Can you work these out from the model? Positions are in its coordinate system, mm. A direction names the side the tool comes from. Round coordinates to 2 decimals unless told otherwise and drop trailing zeros. Loops run counter-clockwise (first coordinate to the right, second up) from the corner with the lowest first, then second, coordinate; pieces in that order, holes last. Notation, with made-up numbers: (1, -18.5) -> (17, -18.5) arc R25 cw to (17, 15.5) -> close; hole circle Ø3 at (30, 18). An arc over 180 degrees is marked (long way). Answer as a JSON object with one key per item and string values.
```python
from build123d import *

# Parameters (mm, degrees)
F0_R      = 36.25
F1_DEPTH  = 17
F2_R      = 32.25
F3_DEPTH  = 4
F4_R      = 1.5
F5_DEPTH  = 15
F7_R      = 2
F8_DEPTH  = 25
F10_R     = 2
F11_DEPTH = 25
F13_DEPTH = 12


with BuildPart() as f1:
    # F0 (on Front) → F1 (new body)
    with BuildSketch(Plane.XZ):
        Circle(F0_R)
        with BuildLine():
            Line((-33, -99), (-18.995849, -99))
            Line((-18.995849, -99), (0, -99))
            Line((0, -99), (18.995849, -99))
            Line((18.995849, -99), (33, -79))
            Line((33, -79), (33, -37.56328))
            ThreePointArc((33, -37.56328), (45.552168, -20.615528), (50, 0))
            ThreePointArc((50, 0), (45.552168, 20.615528), (33, 37.56328))
            Line((33, 37.56328), (33, 79))
            Line((33, 79), (18.995849, 99))
            Line((18.995849, 99), (-18.995849, 99))
            Line((-18.995849, 99), (-33, 99))
            Line((-33, 99), (-33, 79))
            Line((-33, 79), (-33, 37.56328))
            ThreePointArc((-33, 37.56328), (-45.552168, 20.615528), (-50, 0))
            ThreePointArc((-50, 0), (-45.552168, -20.615528), (-33, -37.56328))
            Line((-33, -37.56328), (-33, -79))
            Line((-33, -79), (-33, -99))
        make_face()
        Circle(F0_R, mode=Mode.SUBTRACT)
    extrude(amount=F1_DEPTH)

    # F2 (on face) → F3 (join)
    with BuildSketch(Plane.XZ.offset(17)):
        with BuildLine():
            Line((33, -79), (33, -37.56328))
            ThreePointArc((33, -37.56328), (50, 0), (33, 37.56328))
            Line((33, 37.56328), (33, 79))
            Line((33, 79), (18.995849, 99))
            Line((18.995849, 99), (-33, 99))
            Line((-33, 99), (-33, 37.56328))
            ThreePointArc((-33, 37.56328), (-50, 0), (-33, -37.56328))
            Line((-33, -37.56328), (-33, -99))
            Line((-33, -99), (18.995849, -99))
            Line((18.995849, -99), (33, -79))
        make_face()
        Circle(F2_R, mode=Mode.SUBTRACT)
    extrude(amount=F3_DEPTH)

    # F4 (on face) → F5 (cut)
    with BuildSketch(Plane(origin=(0, 0, 0), x_dir=(-1, 0, 0), z_dir=(0, 1, 0))):
        with Locations((-18, -42.60355)):
            Circle(F4_R)
        with Locations((18, -42.60355)):
            Circle(F4_R)
        with Locations((18, -67.60355)):
            Circle(F4_R)
        with Locations((-18, -67.60355)):
            Circle(F4_R)
    extrude(amount=-F5_DEPTH, mode=Mode.SUBTRACT)

    # F7 (on offset) → F8 (cut)
    with BuildSketch(Plane.YZ.offset(21)):
        with BuildLine():
            ThreePointArc((-12.5, -85.60355), (-10.5, -87.60355), (-8.5, -85.60355))
            Line((-8.5, -85.60355), (-12.5, -85.60355))
        make_face()
        with BuildLine():
            Line((-12.5, -85.60355), (-8.5, -85.60355))
            ThreePointArc((-8.5, -85.60355), (-10.5, -83.60355), (-12.5, -85.60355))
        make_face()
        with BuildLine():
            ThreePointArc((-12.5, -55.10355), (-10.5, -57.10355), (-8.5, -55.10355))
            Line((-8.5, -55.10355), (-12.5, -55.10355))
        make_face()
        with BuildLine():
            Line((-12.5, -55.10355), (-8.5, -55.10355))
            ThreePointArc((-8.5, -55.10355), (-10.5, -53.10355), (-12.5, -55.10355))
        make_face()
        with Locations((-10.5, 55.10355)):
            Circle(F7_R)
        with Locations((-10.5, 85.60355)):
            Circle(F7_R)
    extrude(amount=F8_DEPTH, mode=Mode.SUBTRACT)

    # F10 (on offset) → F11 (cut)
    with BuildSketch(Plane.YZ.offset(-21)):
        with BuildLine():
            ThreePointArc((-12.5, -85.60355), (-10.5, -87.60355), (-8.5, -85.60355))
            Line((-8.5, -85.60355), (-12.5, -85.60355))
        make_face()
        with BuildLine():
            Line((-12.5, -85.60355), (-8.5, -85.60355))
            ThreePointArc((-8.5, -85.60355), (-10.5, -83.60355), (-12.5, -85.60355))
        make_face()
        with BuildLine():
            ThreePointArc((-12.5, -55.10355), (-10.5, -57.10355), (-8.5, -55.10355))
            Line((-8.5, -55.10355), (-12.5, -55.10355))
        make_face()
        with BuildLine():
            Line((-12.5, -55.10355), (-8.5, -55.10355))
            ThreePointArc((-8.5, -55.10355), (-10.5, -53.10355), (-12.5, -55.10355))
        make_face()
        with Locations((-10.5, 55.10355)):
            Circle(F10_R)
        with Locations((-10.5, 85.60355)):
            Circle(F10_R)
    extrude(amount=-F11_DEPTH, mode=Mode.SUBTRACT)

    # F12 (on face) → F13 (cut)
    with BuildSketch(Plane(origin=(0, 0, 0), x_dir=(-1, 0, 0), z_dir=(0, 1, 0))):
        with BuildLine():
            ThreePointArc((0, -87.25), (-2, -89.25), (0, -91.25))
            Line((0, -91.25), (0, -87.25))
        make_face()
        with BuildLine():
            Line((0, -87.25), (0, -91.25))
            ThreePointArc((0, -91.25), (1.414214, -90.664214), (2, -89.25))
            ThreePointArc((2, -89.25), (1.414214, -87.835786), (0, -87.25))
        make_face()
    extrude(amount=-F13_DEPTH, mode=Mode.SUBTRACT)


solid = f1.part
```
Q1. I want a section at D-D, the plane x = 40. Write out the boundary of the cut face in (y, z).
Determined:
{"outline": "(-21, -30) -> (0, -30) -> (0, 30) -> (-21, 30) -> close"}
Q2. I want a section at B-B, the plane z = -20. Write out the boundary of the cut face in (x, y), then the cut area to 3 significant figures.
Determined:
{"outline": "(-45.83, -21) -> (-25.3, -21) -> (-25.3, -17) -> (-30.23, -17) -> (-30.23, 0) -> (-45.83, 0) -> close; (25.3, -21) -> (45.83, -21) -> (45.83, 0) -> (30.23, 0) -> (30.23, -17) -> (25.3, -17) -> close", "area": "694 mm²"}
Q3. I'm going to push flat-ended pins straight in: pin 1 (8 mm diameter, centred on x = 38, y = -4, fed in from -Z); pin 2 (8 mm diameter, centred on y = -9.5, z = 33.5, fed in from -X); pin 3 (0.9 mm diameter, centred on x = 18, z = -68, fed in from +Y). Where does each tip first touch, or does it pass through?
Determined:
{"pin 1": "z = -36.66", "pin 2": "x = -40.37", "pin 3": "y = -15"}
Q4. I want a section at A-A, the plane x = -24. Write out the boundary of the cut face in (y, z), then the cut area to 3 significant figures.
Determined:
{"outline": "(-21, -99) -> (0, -99) -> (0, -27.17) -> (-17, -27.17) -> (-17, -21.54) -> (-21, -21.54) -> close; (-21, 21.54) -> (-17, 21.54) -> (-17, 27.17) -> (0, 27.17) -> (0, 99) -> (-21, 99) -> close; hole circle Ø4 at (-10.5, -85.6); hole circle Ø4 at (-10.5, -55.1); hole circle Ø4 at (-10.5, 55.1); hole circle Ø4 at (-10.5, 85.6)", "area": "3,010 mm²"}
Q5. If I drill on L1, parallel to X at y = -7.5, z = -67.5; L2, parallel to Z at x = 0, y = -19.3; L3, parallel to Z at x = 26.25, y = -10.5, over which ranges is the centre line in solid material (lowest first)? Write a range as [from, to].
Determined:
{"L1": "[-33, -19.5], [-16.5, 16.5], [19.5, 33]", "L2": "[-99, -32.25], [32.25, 99]", "L3": "[-88.64, -87.6], [-83.6, -57.1], [-53.1, -25], [25, 53.1], [57.1, 83.6], [87.6, 88.64]"}
Q6. We'd pull the mould along Y, two halves only. Please class faces 6 (the flat face through (-7, -10, 99)), 7 (the flat face through (0, -12, -89)), 8 (the flat face through (33, -21, 1)), 9 (the cylindrical face through (26.92, -12.09, 53.89)): pulls with the +Y half, pulls with the -Y half, needs draft (parallel to the pull), parting line crosses it, or undercut.
Determined:
{"face 6": "needs draft", "face 7": "pulls with the +Y half", "face 8": "pulls with the -Y half", "face 9": "undercut"}
Q7. On a 3-axis mill with a long thin cutter (end or side, diameter ignored), from which of +Z, -Z, +X, -X, +Y, -Y can I reach the whole of each face in a straight line? I mean faces 1 (the flat face through (-33, -10, 69)), 2 (the flat face through (-33, -10, -68)), 3 (the flat face through (-21, -11, -55)), 4 (the cylindrical face through (34.576, -8.381, 10.889)), 5 (the cylindrical face through (24.36, -10.76, -83.62)). Say none if no direction works.
Determined:
{"face 1": "+Z, -X, +Y, -Y", "face 2": "-Z, -X, +Y, -Y", "face 3": "-X", "face 4": "+Y", "face 5": "+X"}
Q8. I want a section at C-C, the plane x = 9. Write out the boundary of the cut face in (y, z).
Determined:
{"outline": "(-21, -99) -> (0, -99) -> (0, -35.11) -> (-17, -35.11) -> (-17, -30.97) -> (-21, -30.97) -> close; (-21, 30.97) -> (-17, 30.97) -> (-17, 35.11) -> (0, 35.11) -> (0, 99) -> (-21, 99) -> close"}
